Could you check a few things on this model? Use its own coordinates, in mm. A direction names the side the tool comes from. Give positions to 0.01 mm unless a question says otherwise; leave off trailing zeros. Order: outer loops, then holes, each group sorted by start corner. A loop starts at its lowest first (then second) coordinate and runs counter-clockwise, first axis right, second up. Notation, with made-up numbers: M 57.25,17.25 L 71.25,17.25 A19 ccw 71.25,38.25 Z; hole C 78,56.5 d6. An arc over 180 degrees is marked long. Use a Markdown table: item, result. Add a question column.
Item 1: If I drill on L1, parallel to Z at x = 0, y = 27; L2, parallel to Y at x = 0, z = 15; L3, parallel to X at y = -9.5, z = -17, over which ranges is the centre line in solid material (lowest first)? Write a range as from..to.
Item 2: For faces 5 (the face through (9, 15, 0)), 6 (the face through (15, -7, 25)), which set-ups out of +Z, -Z, +X, -X, +Y, -Y let a thin tool reach every point of the face, with its end or its side?
Item 3: Suppose I cut it at C-C on x = 10.5. Write out the boundary of the cut face in (y, z).
Item 4: I'm going to push flat-ended pins straight in: pin 1 Ø1.5 at (y, z) = (3, -7.5) entering from +X; pin 2 Ø8 at (x, z) = (27, -15) entering from -Y; pin 3 Ø1.5 at (y, z) = (-7.5, 18.5) entering from -X. Where does each tip first touch, or does it pass through?
Item 5: Suppose I cut it at D-D on z = -3.5. Write out the boundary of the cut face in (x, y), plus the area to 3 significant figures.
Item 6: Suppose I cut it at B-B on y = 0. Write out the boundary of the cut face in (x, z).
Item 7: If we mould it in two halves opening along X, with no side actions, what happens to faces 1 (the face through (-9, 15, 0)), 2 (the face through (5.668, 24.939, -10.897)), 3 (the face through (-7.5, -33.78, 0.35)), 4 (the face through (15, -7, -25))? For each: released by +X, released by -X, zero draft, split by the parting line, or undercut.
Item 8: Suppose I cut it at A-A on x = 0. Write out the boundary of the cut face in (y, z), plus the area to 3 significant figures.
from build123d import *

# Parameters (mm, degrees)
F0_R          = 34.602453
F0_R_2        = 16.383423
F1_DEPTH      = 25
F1_DEPTH_BACK = 25
F3_R          = 12.283084
F4_DEPTH      = 25


with BuildPart() as f1:
    # F0 (on Top) → F1 (new body, two sides)
    with BuildSketch(Plane.XY) as f1_sk:
        Circle(F0_R)
        Circle(F0_R_2, mode=Mode.SUBTRACT)
    extrude(amount=F1_DEPTH)
    extrude(f1_sk.sketch, amount=-F1_DEPTH_BACK)

    # F3 (on offset) → F4 (cut)
    with BuildSketch(Plane.XZ.offset(-40)):
        Circle(F3_R)
    extrude(amount=F4_DEPTH, mode=Mode.SUBTRACT)


solid = f1.part
Findings below:
| question | item | result |
|---|---|---|
| 1 | L1 | z = -25..-12.28, 12.28..25 |
| 1 | L2 | y = -34.6..-16.38, 16.38..34.6 |
| 1 | L3 | x = -33.27..-13.35, 13.35..33.27 |
| 2 | face 5 | +Y |
| 2 | face 6 | +Z, +X, -X, +Y, -Y |
| 3 | outline | M -32.97,-25 L -12.58,-25 L -12.58,25 L -32.97,25 Z; M 12.58,-25 L 32.97,-25 L 32.97,-6.37 L 15,-6.37 L 15,6.37 L 32.97,6.37 L 32.97,25 L 12.58,25 Z |
| 4 | pin 1 | stops at x = 34.53 |
| 4 | pin 2 | stops at y = -25.85 |
| 4 | pin 3 | stops at x = -33.94 |
| 5 | outline | M -11.77,15 L -11.77,32.54 A34.6 ccw long 11.77,32.54 L 11.77,15 L 6.59,15 A16.38 cw long -6.59,15 Z |
| 5 | area | 2,480 mm^2 |
| 6 | outline | M -34.6,-25 L -16.38,-25 L -16.38,25 L -34.6,25 Z; M 16.38,-25 L 34.6,-25 L 34.6,25 L 16.38,25 Z |
| 7 | face 1 | undercut |
| 7 | face 2 | undercut |
| 7 | face 3 | split by the parting line |
| 7 | face 4 | zero draft |
| 8 | outline | M -34.6,-25 L -16.38,-25 L -16.38,25 L -34.6,25 Z; M 16.38,-25 L 34.6,-25 L 34.6,-12.28 L 16.38,-12.28 Z; M 16.38,12.28 L 34.6,12.28 L 34.6,25 L 16.38,25 Z |
| 8 | area | 1,370 mm^2 |
